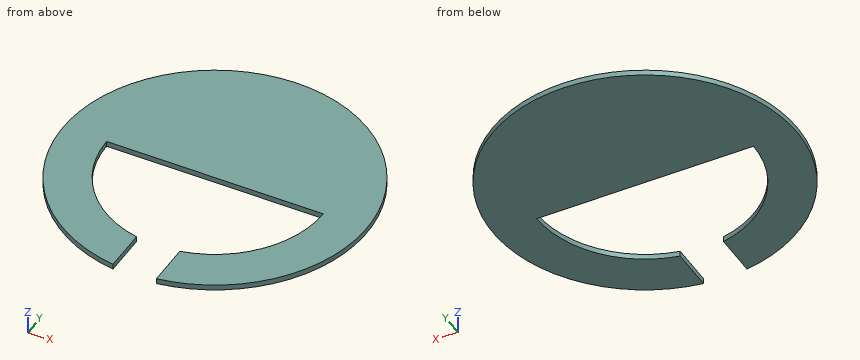
from build123d import *

# Parameters (mm, degrees)
F0_R     = 88.9
F1_DEPTH = 3.175
F3_DEPTH = 6.35


with BuildPart() as f1:
    # F0 (on Top) → F1 (new body)
    with BuildSketch(Plane.XY):
        Circle(F0_R)
        with BuildLine():
            ThreePointArc((-63.5, 0), (0, 63.5), (63.5, 0))
            ThreePointArc((63.5, 0), (0, -63.5), (-63.5, 0))
        make_face(mode=Mode.SUBTRACT)
        with BuildLine():
            Line((-63.5, 0), (63.5, 0))
            ThreePointArc((63.5, 0), (0, 63.5), (-63.5, 0))
        make_face()
    extrude(amount=F1_DEPTH)

    # F2 (on face) → F3 (cut)
    with BuildSketch(Plane.XY.offset(3.175)):
        Polygon((12.7, -58.594692), (0, -58.594692), (-12.7, -58.594692), (-12.7, -96.489258), (12.7, -96.489258), align=None)
    extrude(amount=-F3_DEPTH, mode=Mode.SUBTRACT)


solid = f1.part
Input: part model. Units: mm. Frame: model coordinates. Give positions to 0.01 mm unless a question says otherwise; leave off trailing zeros. Order: outer loops, then holes, each group sorted by start corner. A loop starts at its lowest first (then second) coordinate and runs counter-clockwise, first axis right, second up. Notation, with made-up numbers: (29, 5) -> (79, 5) arc R14 cw to (79, 9) -> close; hole circle Ø2 at (47, 49.5). An arc over 180 degrees is marked (long way). Use one line per item in the form item = value.
1) First-contact query: pin 1 Ø1.5 at (y, z) = (-46.5, 2.5) entering from +X; pin 2 Ø1.5 at (y, z) = (68.5, 1) entering from +X; pin 3 Ø1 at (x, z) = (23, 1.5) entering from -Y. Flat tips, straight axial feed; report the tip coordinate or a pass-through.
Response values:
pin_1 = 76.22
pin_2 = 57.56
pin_3 = -86.01
2) Section D-D, the plane y = 44. Return loops of the section in (x, z) (3 decimals).
Response values:
outline = (-77.248, 0) -> (77.248, 0) -> (77.248, 3.175) -> (-77.248, 3.175) -> close
3) Section B-B, the plane z = 1.55. Return loops of the section in (x, y), and give its area (3 significant figures).
Response values:
outline = (-63.5, 0) -> (63.5, 0) arc R63.5 cw to (12.7, -62.22) -> (12.7, -87.99) arc R88.9 ccw (long way) to (-12.7, -87.99) -> (-12.7, -62.22) arc R63.5 cw to start
area = 17,800 mm^2
4) Section C-C, the plane x = 0. Return loops of the section in (y, z) (3 decimals), and give its area (3 significant figures).
Response values:
outline = (0, 0) -> (88.9, 0) -> (88.9, 3.175) -> (0, 3.175) -> close
area = 282 mm^2
5) Section A-A, the plane y = -28. Return loops of the section in (x, z) (3 decimals).
Response values:
outline = (-84.375, 0) -> (-56.993, 0) -> (-56.993, 3.175) -> (-84.375, 3.175) -> close; (56.993, 0) -> (84.375, 0) -> (84.375, 3.175) -> (56.993, 3.175) -> close
6) Line query: probe 1 along X at (y, z) = (-0.5, 0.75); probe 2 along Y at (x, z) = (41, 2.95); probe 3 along Y at (x, z) = (-30.5, 1.25). Output: solid intervals per line, ascending.
Response values:
probe_1 = -88.9 to -63.5, 63.5 to 88.9
probe_2 = -78.88 to -48.49, 0 to 78.88
probe_3 = -83.5 to -55.7, 0 to 83.5
